Source: CAD feature listing. Evaluate the final solid. Frame: model axes, mm. A direction names the side the tool comes from. Give positions to 0.01 mm unless a question says otherwise; leave off trailing zeros. Write each loop counter-clockwise with the first axis right and the second up, starting at its lowest first coordinate (ties: lowest second). Pieces come first, ordered by that corner, then holes. Notation, with made-up numbers: (82.5, -25) -> (137.5, -25) arc R18 ccw to (137.5, -15) -> close; hole circle Ø4 at (50.5, 85). An arc over 180 degrees is marked (long way). Write item = value, one per line.
from build123d import *

# Parameters (mm, degrees)
IZIM1_W                     = 130
IZIM1_H                     = 160
Y_KSEKLIK_EKSTR_ZYON1_DEPTH = 4
IZIM3_W                     = 55
IZIM3_H                     = 25
KES_EKSTR_ZYON1_DEPTH       = 4
KES_EKSTR_ZYON2_DEPTH       = 10
IZIM5_W                     = 54.012242348
IZIM5_H                     = 68.899562137
KES_EKSTR_ZYON3_DEPTH       = 2
IZIM8_W                     = 54.469692937
IZIM8_H                     = 69.59441616
KES_EKSTR_ZYON5_DEPTH       = 2
IZIM9_R                     = 1.5
KES_EKSTR_ZYON6_DEPTH       = 5
IZIM10_W                    = 27
IZIM10_H                    = 34.5
KES_EKSTR_ZYON7_DEPTH       = 2
IZIM11_R                    = 1.5
KES_EKSTR_ZYON8_DEPTH       = 5
KES_EKSTR_ZYON9_DEPTH       = 104.155222988
KES_EKSTR_ZYON9_DEPTH_BACK  = 5
KES_EKSTR_ZYON10_DEPTH      = 2
IZIM14_W                    = 5
IZIM14_H                    = 5.1
KES_EKSTR_ZYON11_DEPTH      = 9
IZIM15_W                    = 6.934142085
IZIM15_H                    = 14.276174882
IZIM15_W_2                  = 19.374808768
IZIM15_H_2                  = 6.934142085
KES_EKSTR_ZYON12_DEPTH      = 9
IZIM16_R                    = 1.5
KES_EKSTR_ZYON13_DEPTH      = 10
IZIM17_W                    = 7.6
IZIM17_H                    = 8.3
KES_EKSTR_ZYON14_DEPTH      = 10


with BuildPart() as part:
    # Çizim1 → Yükseklik-Ekstrüzyon1 (new body)
    with BuildSketch(Plane.XY):
        Rectangle(IZIM1_W, IZIM1_H)
    extrude(amount=Y_KSEKLIK_EKSTR_ZYON1_DEPTH)

    # Çizim3 → Kes-Ekstrüzyon1 (cut)
    with BuildSketch(Plane(origin=(0, 0, 0), x_dir=(-1, 0, 0), z_dir=(0, 0, -1))):
        with Locations((37.5, 67.5)):
            Rectangle(IZIM3_W, IZIM3_H)
        with Locations((-37.5, 67.5)):
            Rectangle(IZIM3_W, IZIM3_H)
    extrude(amount=-KES_EKSTR_ZYON1_DEPTH, mode=Mode.SUBTRACT)

    # Çizim4 → Kes-Ekstrüzyon2 (cut)
    with BuildSketch(Plane.XY.offset(4)):
        with BuildLine():
            Line((-24.249382275, -27.006425474), (24.249382275, -27.006425474))
            add(Edge.make_bspline(
                [(65, -43.244851104), (59.485167295, -111.431741319), (24.249382275, -27.006425474)],
                knots=[0, 0, 0, 1, 1, 1], degree=2))
            Line((65, -43.244851104), (65, -80))
            Line((65, -80), (-65, -80))
            Line((-65, -80), (-65, -43.244851104))
            add(Edge.make_bspline(
                [(-65, -43.244851104), (-59.485167295, -111.431741319), (-24.249382275, -27.006425474)],
                knots=[0, 0, 0, 1, 1, 1], degree=2))
        make_face()
    extrude(amount=-KES_EKSTR_ZYON2_DEPTH, mode=Mode.SUBTRACT)

    # Çizim5 → Kes-Ekstrüzyon3 (cut)
    with BuildSketch(Plane.XY.offset(4)):
        with Locations((-1.54185026, 8.138209618)):
            Rectangle(IZIM5_W, IZIM5_H)
    extrude(amount=-KES_EKSTR_ZYON3_DEPTH, mode=Mode.SUBTRACT)

    # Çizim8 → Kes-Ekstrüzyon5 (cut)
    with BuildSketch(Plane.XY.offset(4)):
        with Locations((-1.313124966, 7.790782606)):
            Rectangle(IZIM8_W, IZIM8_H)
    extrude(amount=-KES_EKSTR_ZYON5_DEPTH, mode=Mode.SUBTRACT)

    # Çizim9 → Kes-Ekstrüzyon6 (cut)
    with BuildSketch(Plane.XY.offset(4)):
        with Locations((-10.095729086, 39.728428549)):
            Circle(IZIM9_R)
        with Locations((17.844270914, 39.728428549)):
            Circle(IZIM9_R)
        with Locations((-25.335729086, -11.071571451)):
            Circle(IZIM9_R)
        with Locations((22.924270914, -12.341571451)):
            Circle(IZIM9_R)
    extrude(amount=-KES_EKSTR_ZYON6_DEPTH, mode=Mode.SUBTRACT)

    # Çizim10 → Kes-Ekstrüzyon7 (cut)
    with BuildSketch(Plane.XY.offset(4)):
        with Locations((-48, -6.037117551)):
            Rectangle(IZIM10_W, IZIM10_H)
        with Locations((48, -6.037117551)):
            Rectangle(IZIM10_W, IZIM10_H)
    extrude(amount=-KES_EKSTR_ZYON7_DEPTH, mode=Mode.SUBTRACT)

    # Çizim11 → Kes-Ekstrüzyon8 (cut)
    with BuildSketch(Plane.XY.offset(4)):
        with Locations((-57.85, -19.637117551)):
            Circle(IZIM11_R)
        with Locations((-38.15, -19.637117551)):
            Circle(IZIM11_R)
        with Locations((-38.15, 6.562882449)):
            Circle(IZIM11_R)
        with Locations((-57.85, 6.562882449)):
            Circle(IZIM11_R)
        with Locations(Location((57.85, -19.637117551, 0), (0, 0, 180))):
            Circle(IZIM11_R)
        with Locations(Location((38.15, -19.637117551, 0), (0, 0, 180))):
            Circle(IZIM11_R)
        with Locations(Location((38.15, 6.562882449, 0), (0, 0, 180))):
            Circle(IZIM11_R)
        with Locations(Location((57.85, 6.562882449, 0), (0, 0, 180))):
            Circle(IZIM11_R)
    extrude(amount=-KES_EKSTR_ZYON8_DEPTH, mode=Mode.SUBTRACT)

    # Çizim12 → Kes-Ekstrüzyon9 (cut, two sides)
    with BuildSketch(Plane.XY.offset(4)) as kes_ekstr_zyon9_sk:
        with BuildLine():
            Line((-65, 55), (-65, 21.312671553))
            add(Edge.make_bspline(
                [(-65, 21.312671553), (-63.962297288, 53.139320322), (-23.182224936, 55)],
                knots=[0, 0, 0, 0.889532369, 0.889532369, 0.889532369], degree=2))
            Line((-23.182224936, 55), (-65, 55))
        make_face()
        with BuildLine():
            add(Edge.make_bspline(
                [(65, 21.312671553), (63.962297288, 53.139320322), (23.182224936, 55)],
                knots=[0, 0, 0, 0.889532369, 0.889532369, 0.889532369], degree=2))
            Line((65, 21.312671553), (65, 55))
            Line((65, 55), (23.182224936, 55))
        make_face()
    extrude(amount=KES_EKSTR_ZYON9_DEPTH, mode=Mode.SUBTRACT)
    extrude(kes_ekstr_zyon9_sk.sketch, amount=-KES_EKSTR_ZYON9_DEPTH_BACK, mode=Mode.SUBTRACT)

    # Çizim13 → Kes-Ekstrüzyon10 (cut)
    with BuildSketch(Plane.XY.offset(4)):
        Polygon((0, 50), (0, 80), (-10, 80), (-10, 55), (-10, 50), align=None)
        Polygon((10, 80), (0, 80), (0, 50), (10, 50), (10, 55), align=None)
    extrude(amount=-KES_EKSTR_ZYON10_DEPTH, mode=Mode.SUBTRACT)

    # Çizim14 → Kes-Ekstrüzyon11 (cut)
    with BuildSketch(Plane.XY.offset(2)):
        with Locations((-2.5, 52.55)):
            Rectangle(IZIM14_W, IZIM14_H)
        with Locations((2.5, 52.55)):
            Rectangle(IZIM14_W, IZIM14_H)
    extrude(amount=-KES_EKSTR_ZYON11_DEPTH, mode=Mode.SUBTRACT)

    # Çizim15 → Kes-Ekstrüzyon12 (cut)
    with BuildSketch(Plane.XY.offset(4)):
        with Locations((-39.157508247, 36.812518567)):
            Rectangle(IZIM15_W, IZIM15_H)
        with Locations((-47.213349787, 18.865327288)):
            Rectangle(IZIM15_W_2, IZIM15_H_2)
        with Locations((39.157508247, 36.812518567)):
            Rectangle(IZIM15_W, IZIM15_H)
        with Locations((47.213349787, 18.865327288)):
            Rectangle(IZIM15_W_2, IZIM15_H_2)
    extrude(amount=-KES_EKSTR_ZYON12_DEPTH, mode=Mode.SUBTRACT)

    # Çizim16 → Kes-Ekstrüzyon13 (cut)
    with BuildSketch(Plane.XY.offset(2)):
        with Locations((-17.844270914, 39.728428549)):
            Circle(IZIM16_R)
    extrude(amount=-KES_EKSTR_ZYON13_DEPTH, mode=Mode.SUBTRACT)

    # Çizim17 → Kes-Ekstrüzyon14 (cut)
    with BuildSketch(Plane.XY.offset(2)):
        with Locations((-3.8, 36.638150808)):
            Rectangle(IZIM17_W, IZIM17_H)
        with Locations((3.8, 36.638150808)):
            Rectangle(IZIM17_W, IZIM17_H)
    extrude(amount=-KES_EKSTR_ZYON14_DEPTH, mode=Mode.SUBTRACT)


solid = part.part
(1) Section query B-B (y = -3.5). Return loops of the section in (x, z), plus the area to 3 significant figures.
Values follow:
outline = (-65, 0) -> (65, 0) -> (65, 4) -> (61.5, 4) -> (61.5, 2) -> (34.5, 2) -> (34.5, 4) -> (25.92, 4) -> (25.92, 2) -> (-28.55, 2) -> (-28.55, 4) -> (-34.5, 4) -> (-34.5, 2) -> (-61.5, 2) -> (-61.5, 4) -> (-65, 4) -> close
area = 303 mm2
(2) First-contact query: pin 1 (2 mm diameter, centred on x = 49, z = 2, fed in from +Y); pin 2 (2 mm diameter, centred on y = 33.5, z = 2.5, fed in from +X); pin 3 (10 mm diameter, centred on x = -2, y = 68.5, fed in from +Z); pin 4 (5 mm diameter, centred on x = -38.15, y = -19.64, fed in from -Z). Flat tips, straight axial feed; report the tip coordinate or a pass-through.
Values follow:
pin_1 = 49.48
pin_2 = 63.11
pin_3 = 2
pin_4 = 0
(3) Access query for faces 1 (the face through (-16, 55, 2)), 2 (the face through (-48, -6, 2)), 3 (the face through (-30, -9, 4)), 4 (the face through (47, 22.332, 2)). Directions: +Z, -Z, +X, -X, +Y, -Y. A direction counts if a zero-diameter tool reaches every point of the face in a straight line with its end or side. Return the directions, or none.
Values follow:
face_1 = +Z, -Z, -X, +Y
face_2 = +Z
face_3 = +Z, +X, -X, +Y, -Y
face_4 = +Z, -Z
(4) Section query C-C (z = 3.05). Give the number of separate pieces and of enclosed holes in the cut face, plus the area to 3 significant figures.
Values follow:
separate_pieces = 1
enclosed_holes = 6
area = 6,470 mm2
(5) Material intervals for line 1 (Y direction, x = -1.5, z = 0.75); line 2 (X direction, y = 7, z = 2.5); line 3 (Y direction, x = 38.15, z = 1.35), sorted ascending.
Values follow:
line_1 = -27.01 to 32.49, 40.79 to 50, 55.1 to 80
line_2 = -65 to -61.5, -34.5 to -28.55, 25.92 to 34.5, 61.5 to 65
line_3 = -56.47 to -21.14, -18.14 to 5.06, 8.06 to 15.4, 22.33 to 29.67, 43.95 to 53
(6) Pull-direction query (X, two-part tool) for faces 5 (the face through (0, 50, 2)), 6 (the face through (65, -11, 2)), 7 (the face through (-65, -11, 2)), 8 (the face through (35.69, 37, 2)); classes: pulls with the +X half, pulls with the -X half, needs draft (parallel to the pull), parting line crosses it, or undercut.
Values follow:
face_5 = undercut
face_6 = pulls with the +X half
face_7 = pulls with the -X half
face_8 = undercut
(7) Section query A-A (y = 19.5). Return loops of the section in (x, z), plus the area to 3 significant figures.
Values follow:
outline = (-65, 0) -> (-56.9, 0) -> (-56.9, 4) -> (-65, 4) -> close; (-37.53, 0) -> (37.53, 0) -> (37.53, 4) -> (25.92, 4) -> (25.92, 2) -> (-28.55, 2) -> (-28.55, 4) -> (-37.53, 4) -> close; (56.9, 0) -> (65, 0) -> (65, 4) -> (56.9, 4) -> close
area = 256 mm2
